```python
from build123d import *

# Parameters (mm, degrees)
F0_W         = 80.7386888191
F0_H         = 76.366558671
F1_DEPTH     = 9.144
F2_W         = 55.6718036532
F2_H         = 9.6186883748
F3_DEPTH     = 70.358
F4_W         = 9.0357391164
F4_H         = 76.0750807822
F5_DEPTH     = 55.626
F6_SIZE      = 45.72
F7_T1_DEPTH  = 167.084926268
F8_T1_DEPTH  = 193.8162932759
F9_T4_DEPTH  = 127.8865685488
F10_T4_DEPTH = 246.7691481608
F12_DEPTH    = 44.958
F14_DEPTH    = 35.306
F15_R        = 6.35
F15_R_2      = 7.0169538455
F16_DEPTH    = 55.372


# Not quite as in the source:
# - a fillet or chamfer that OpenCascade refuses, or shapes differently, is made with other operations: its cross-section is extruded or revolved along the edge and cut away or added


with BuildPart() as f1:
    # F0 (on Front) → F1 (new body)
    with BuildSketch(Plane.XZ):
        with Locations((-31.0421311297, 2.4775415659)):
            Rectangle(F0_W, F0_H)
        with BuildLine():
            Line((-60.626886785, -8.890000172), (-60.626886785, 15.8854108304))
            ThreePointArc((-60.626886785, 15.8854108304), (-54.5059032738, 22.0063943416), (-48.3849197626, 15.8854108304))
            Line((-48.3849197626, 15.8854108304), (-48.3849197626, -8.890000172))
            ThreePointArc((-48.3849197626, -8.890000172), (-54.5059032738, -15.0109836832), (-60.626886785, -8.890000172))
        make_face(mode=Mode.SUBTRACT)
        with BuildLine():
            Line((-34.9770486355, -8.890000172), (-34.9770486355, 15.8854108304))
            ThreePointArc((-34.9770486355, 15.8854108304), (-28.8560651243, 22.0063943416), (-22.7350816131, 15.8854108304))
            Line((-22.7350816131, 15.8854108304), (-22.7350816131, -8.890000172))
            ThreePointArc((-22.7350816131, -8.890000172), (-28.8560651243, -15.0109836832), (-34.9770486355, -8.890000172))
        make_face(mode=Mode.SUBTRACT)
        Polygon((70.5370530486, -35.7057377696), (9.3272132799, 40.6608209014), (9.3272132799, -35.7057377696), align=None)
    extrude(amount=F1_DEPTH)

    # F2 (on Right) → F3 (join)
    with BuildSketch(Plane.YZ):
        with Locations((-27.8359018266, -40.2236077935)):
            Rectangle(F2_W, F2_H)
    extrude(amount=F3_DEPTH)

    # F4 (on Front) → F5 (join)
    with BuildSketch(Plane.XZ):
        with Locations((4.5178695582, 2.9147546738)):
            Rectangle(F4_W, F4_H)
    extrude(amount=F5_DEPTH)

    # F6
    f6_edges = [f1.edges().sort_by_distance(p)[0] for p in [
        (4.51787, -55.626, 40.952295),
    ]]
    chamfer(f6_edges, length=F6_SIZE)

    # F7: chamfer of 30.48 on 1 edges, made by hand

    # F7_s2 → F7_t1 (cut)
    with BuildSketch(Plane.YZ.offset(-79.0245935758)):
        Polygon((-34.0733853094, 16.7849097555), (-55.626, -35.2477049351), (-55.626, -4.7677049351), align=None)
    extrude(amount=F7_T1_DEPTH, mode=Mode.SUBTRACT)

    # F8: chamfer of 35.56 on 1 edges, made by hand

    # F8_s2 → F8_t1 (cut)
    with BuildSketch(Plane.YZ.offset(-92.3902770798)):
        Polygon((-8.9286681704, 41.9296268945), (-47.6816081643, -16.0682464206), (-34.0733853094, 16.7849097555), align=None)
    extrude(amount=F8_T1_DEPTH, mode=Mode.SUBTRACT)

    # F9: chamfer of 22.86 on 1 edges, made by hand


with BuildPart() as f9_tool2:
    # F9_s3 → F9_t4 (new body)
    with BuildSketch(Plane.YZ.offset(-59.4254147162)):
        Polygon((-34.9812726375, 2.9391489166), (-56.4297514282, -37.1881325338), (-47.6816081643, -16.0682464206), align=None)
    extrude(amount=F9_T4_DEPTH)

    split(bisect_by=Plane.XY.offset(-35.4142636061), keep=Keep.TOP)


with BuildPart() as f1_1:
    add(f1.part)

    # F9_t1: cut F9_tool2
    add(f9_tool2.part, mode=Mode.SUBTRACT)

    # F10: chamfer of 45.72 on 1 edges, made by hand


with BuildPart() as f10_tool2:
    # F10_s3 → F10_t4 (new body)
    with BuildSketch(Plane.YZ.offset(-118.8667045222)):
        Polygon((-56.5335314452, -37.3822912894), (-9.5806015838, 40.9539395911), (-34.9812726375, 2.9391489166), align=None)
    extrude(amount=F10_T4_DEPTH)

    split(bisect_by=Plane.XY.offset(-35.1227857172), keep=Keep.TOP)


with BuildPart() as f1_2:
    add(f1_1.part)

    # F10_t1: cut F10_tool2
    add(f10_tool2.part, mode=Mode.SUBTRACT)

    # F11 (on Top) → F12 (join)
    with BuildSketch(Plane.XY):
        Polygon((-70.8285272121, -16.7598351836), (0, -55.2345886827), (0, -9.472951293), (-70.8285272121, -9.472951293), align=None)
    extrude(amount=-F12_DEPTH)

    # F13 (on Top) → F14 (cut)
    with BuildSketch(Plane.XY):
        Polygon((0, -9.1814752668), (-71.4114755392, -9.1814752668), (-71.4114755392, -16.4683610201), (0, -55.8175444603), align=None)
    extrude(amount=-F14_DEPTH, mode=Mode.SUBTRACT)

    # F15 (on Top) → F16 (cut)
    with BuildSketch(Plane.XY):
        with Locations((24.775644736, -30.7506565005)):
            Circle(F15_R)
        with Locations((49.3974882285, -30.7506565005)):
            Circle(F15_R_2)
    extrude(amount=-F16_DEPTH, mode=Mode.SUBTRACT)


solid = f1_2.part
```
Work out the finished part from the listing and answer in its coordinate system (mm). A direction names the side the tool comes from. Give positions to 0.01 mm unless a question says otherwise; leave off trailing zeros. Order: outer loops, then holes, each group sorted by start corner. A loop starts at its lowest first (then second) coordinate and runs counter-clockwise, first axis right, second up. Notation, with made-up numbers: M 36.5,75.5 L 58.5,75.5 A26 cw 58.5,113.5 Z; hole C -37,59.25 d8. An arc over 180 degrees is marked long. Return JSON: item names as keys, results as strings.
1) Section D-D, the plane x = 33 is taken. Write down the section's boundary in (y, z).
Resolved:
{"outline": "M -55.67,-45.03 L 0,-45.03 L 0,11.13 L -9.14,11.13 L -9.14,-35.41 L -55.67,-35.41 Z"}
2) Section B-B, the plane z = 3 is taken. Write down the section's boundary in (x, y), plus the area to 4 significant figures.
Resolved:
{"outline": "M -71.41,-9.14 L -60.63,-9.14 L -60.63,0 L -71.41,0 Z; M -48.38,-9.14 L -34.98,-9.14 L -34.98,0 L -48.38,0 Z; M -22.74,-9.14 L 0,-9.14 L 0,-32.33 L 9.04,-32.33 L 9.04,-9.14 L 39.51,-9.14 L 39.51,0 L -22.74,0 Z", "area": "1,000 mm^2"}
3) For a pull along X with two mould halves and no side action, classify faces 1 (the flat face through (-17, -9.144, -5)), 2 (the flat face through (40.242, -4.508, 2.091)), 3 (the cylindrical face through (-54.64, -4.508, 22.005)) as +X half, -X half, draft (parallel to the pull), parting line (faces both ways), or undercut.
Resolved:
{"face 1": "draft", "face 2": "+X half", "face 3": "undercut"}
4) A tool of negligible diameter and unlimited length cuts with its end or side. For faces 4 (the flat face through (-36, -5, -35.706)), 5 (the flat face through (-22.735, -5, 4)), 6 (the flat face through (-28, -27, -35.306)), from which of +Z, -Z, +X, -X, +Y, -Y can it reach the whole face along a straight path? Write none if from no direction.
Resolved:
{"face 4": "-Z, -X, +Y", "face 5": "+Y, -Y", "face 6": "+Z, +X, -X, -Y"}
5) Section C-C, the plane x = -19.5 is taken. Write down the section's boundary in (y, z), plus the area to 3 significant figures.
Resolved:
{"outline": "M -44.64,-44.96 L -9.47,-44.96 L -9.47,-35.31 L -44.64,-35.31 Z; M -9.14,-35.71 L 0,-35.71 L 0,40.66 L -9.14,40.66 Z", "area": "1,040 mm^2"}
6) Straight lines are drawn through the part: line 1 along Z through (x, y) = (-23.5, -42); line 2 along Z through (x, y) = (14, -14); line 3 along Y through (x, z) = (-15.5, -22.5). For each, find the intervals that lie inside material, in ascending order. Write a range as [from, to].
Resolved:
{"line 1": "[-44.96, -35.31]", "line 2": "[-45.03, -35.41]", "line 3": "[-9.14, 0]"}
7) Each of these flat-tipped pins is pushed along its axis until it touches: pin 1 (10.5 mm diameter, centred on y = -28, z = -41.5, fed in from -X); pin 2 (2.5 mm diameter, centred on x = -43.5, y = -3, fed in from -Z); pin 3 (4 mm diameter, centred on x = 32.5, z = -26.5, fed in from -Y). Where does it stop, or does it pass through?
Resolved:
{"pin 1": "x = -59.8", "pin 2": "z = -35.71", "pin 3": "y = -9.14"}
8) Section A-A, the plane y = -32.5 is taken. Write down the section's boundary in (x, z).
Resolved:
{"outline": "M -41.85,-44.96 L 0,-44.96 L 0,-45.03 L 18.67,-45.03 L 18.67,-35.41 L 0,-35.41 L 0,-35.31 L -41.85,-35.31 Z; M 0,-35.12 L 9.04,-35.12 L 9.04,2.72 L 0,2.72 Z; M 30.88,-45.03 L 42.6,-45.03 L 42.6,-35.41 L 30.88,-35.41 Z; M 56.19,-45.03 L 70.36,-45.03 L 70.36,-35.41 L 56.19,-35.41 Z"}
